Part model, mm, in its own coordinate system. A direction names the side the tool comes from. Coordinates: 2 decimals unless noted, no trailing zeros. Loops run counter-clockwise (first coordinate to the right, second up) from the corner with the lowest first, then second, coordinate; pieces in that order, holes last. Notation, with made-up numbers: M 29.25,26.25 L 73.25,26.25 A22 ccw 73.25,36.25 Z; hole C 60,7.5 d10. An arc over 180 degrees is marked long. Use a Markdown table: item, result. Add a question column.
1) Band-saw the part on D-D (y = -35.5). List the corners of the cut face in (x, z).
2) Band-saw the part on B-B (x = 6.5). List the corners of the cut face in (y, z), plus the area to 3 significant figures.
3) Pin check, flat tips, straight feed: pin 1 Ø3 at (x, y) = (1.5, -34) entering from +Z; pin 2 Ø1 at (x, z) = (10, 1) entering from -Y; pin 3 Ø1 at (x, z) = (17, 1.5) entering from +Y; pin 4 Ø1 at (y, z) = (-41, 1) entering from +X. Stop position of each tip, or through.
4) Band-saw the part on A-A (z = 0.4). List the corners of the cut face in (x, y) (3 decimals), plus the area to 3 significant figures.
5) Wall check: probe 1 along X at (y, z) = (-29.25, 1.9); probe 2 along Y at (x, z) = (29.5, 1.5); probe 3 along Y at (x, z) = (31, 0.95). Give the ranges that are in metal, low to high. Write a range as from..to.
6) Band-saw the part on C-C (y = -43.25). List the corners of the cut face in (x, z).
7) Tool access for faces 1 (the flat face through (15, -35, 2)), 2 (the flat face through (20.772, -29.133, 0.986)): list every direction of +Z, -Z, +X, -X, +Y, -Y with a clear straight run to the whole face (end or side of a thin tool).
from build123d import *

# Parameters (mm, degrees)
SKETCH_1_R      = 2
SKETCH_1_R_2    = 1.25
EXTRUDE_1_DEPTH = 2


with BuildPart() as part:
    # 草图1 → 凸台-拉伸1 (new body)
    with BuildSketch(Plane.XY):
        with BuildLine():
            Line((12.667014152, -29.085004895), (0.259047619, -37.62952381))
            ThreePointArc((0.259047619, -37.62952381), (-3.602527799, -40.586338642), (-1.755121481, -45.085406162))
            ThreePointArc((-1.755121481, -45.085406162), (17.862485508, -41.627982305), (34.178996295, -30.201007228))
            ThreePointArc((34.178996295, -30.201007228), (32.303988677, -25.71337254), (27.482658695, -26.353134885))
            Line((27.482658695, -26.353134885), (13.870853157, -31.991329347))
            Line((13.870853157, -31.991329347), (12.667014152, -29.085004895))
        make_face()
        with Locations((0.259047619, -41.62952381)):
            Circle(SKETCH_1_R, mode=Mode.SUBTRACT)
        with Locations((30.311085819, -29.18156201)):
            Circle(SKETCH_1_R, mode=Mode.SUBTRACT)
        with Locations((5.724004276, -40.783180011)):
            Circle(SKETCH_1_R_2, mode=Mode.SUBTRACT)
    extrude(amount=EXTRUDE_1_DEPTH)


solid = part.part
Entries:
| question | item | result |
|---|---|---|
| 1 | outline | M 3.35,0 L 28.42,0 L 28.42,2 L 3.35,2 Z |
| 2 | outline | M -44.7,0 L -41.76,0 L -41.76,2 L -44.7,2 Z; M -39.8,0 L -33.33,0 L -33.33,2 L -39.8,2 Z |
| 2 | area | 18.8 mm2 |
| 3 | pin 1 | through |
| 3 | pin 2 | y = -44.19 |
| 3 | pin 3 | y = -30.49 |
| 3 | pin 4 | x = 20.37 |
| 4 | outline | M -1.755,-45.085 A46 ccw 34.179,-30.201 A4 ccw 27.483,-26.353 L 13.871,-31.991 L 12.667,-29.085 L 0.259,-37.63 A4 ccw Z; hole C 0.259,-41.63 d4; hole C 5.724,-40.783 d2.5; hole C 30.311,-29.182 d4 |
| 4 | area | 349 mm2 |
| 5 | probe 1 | 12.43..12.74, 20.49..28.31, 32.31..34.31 |
| 5 | probe 2 | -34.64..-31.01, -27.35..-25.26 |
| 5 | probe 3 | -33.35..-31.06, -27.3..-25.24 |
| 6 | outline | M -3.4,0 L -0.91,0 L -0.91,2 L -3.4,2 Z; M 1.43,0 L 13.27,0 L 13.27,2 L 1.43,2 Z |
| 7 | face 1 | +Z, +X, -X, +Y, -Y |
| 7 | face 2 | +Z, -Z, +Y |
